Input: dimensioned drawing with shaded views. Units: mm. Origin: part minimum x, y, z. A direction names the side the tool comes from. Round coordinates to 2 decimals unless told otherwise and drop trailing zeros. Loops run counter-clockwise (first coordinate to the right, second up) from the corner with the lowest first, then second, coordinate; pieces in that order, holes last. Notation, with made-up numbers: M 39,-32 L 80,-32 A25 cw 80,0 Z; hole C 23.25,-11.75 d11. An arc over 180 degrees is marked long. Answer as a JSON object with one key per item and string values.
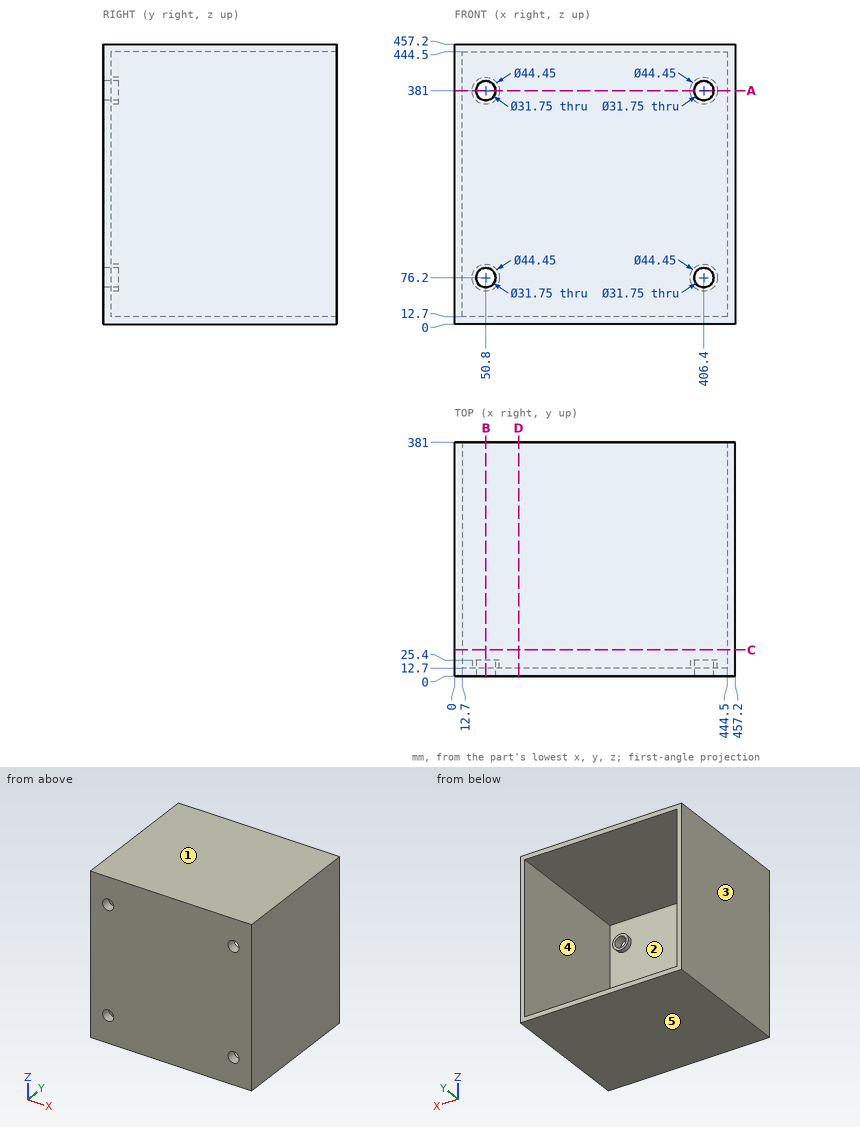
Item 1: Access query for the marked faces 1 and 2. Directions: +Z, -Z, +X, -X, +Y, -Y. A direction counts if a zero-diameter tool reaches every point of the face in a straight line with its end or side. Return the directions, or none.
Answer sheet:
{"face 1": "+Z, +X, -X, +Y, -Y", "face 2": "+Y"}
Item 2: Section B-B on x = 50.8. Return the cut outline in (y, z) (3 decimals), then the cut area to 3 significant figures.
Answer sheet:
{"outline": "M 0,0 L 381,0 L 381,12.7 L 12.7,12.7 L 12.7,53.975 L 25.4,53.975 L 25.4,60.325 L 0,60.325 Z; M 0,92.075 L 25.4,92.075 L 25.4,98.425 L 12.7,98.425 L 12.7,358.775 L 25.4,358.775 L 25.4,365.125 L 0,365.125 Z; M 0,396.875 L 25.4,396.875 L 25.4,403.225 L 12.7,403.225 L 12.7,444.5 L 381,444.5 L 381,457.2 L 0,457.2 Z", "area": "14,700 mm²"}
Item 3: Pull-direction query (X, two-part tool) for the marked faces 3, 4 and 5; classes: pulls with the +X half, pulls with the -X half, needs draft (parallel to the pull), parting line crosses it, or undercut.
Answer sheet:
{"face 3": "pulls with the -X half", "face 4": "undercut", "face 5": "needs draft"}
Item 4: Line query: probe 1 along Z at (x, y) = (406, 16); probe 2 along X at (y, z) = (11.75, 381) (3 decimals); probe 3 along X at (y, z) = (18, 381) (3 decimals). Output: solid intervals per line, ascending. Write a range as from..to.
Answer sheet:
{"probe 1": "z = 0..12.7, 53.98..60.33, 92.07..98.42, 358.78..365.13, 396.87..403.22, 444.5..457.2", "probe 2": "x = 0..34.925, 66.675..390.525, 422.275..457.2", "probe 3": "x = 0..12.7, 28.575..34.925, 66.675..73.025, 384.175..390.525, 422.275..428.625, 444.5..457.2"}
Item 5: Contact query for flat-ended pins moving along their axis: pin 1 Ø8 at (x, z) = (285.5, 287.5) entering from +Y; pin 2 Ø13.5 at (x, z) = (398.5, 66) entering from +Y. Output: stop coordinate, or through.
Answer sheet:
{"pin 1": "stops at y = 12.7", "pin 2": "stops at y = 25.4"}
Item 6: Section D-D on x = 104.5. Return the cut outline in (y, z).
Answer sheet:
{"outline": "M 0,0 L 381,0 L 381,12.7 L 12.7,12.7 L 12.7,444.5 L 381,444.5 L 381,457.2 L 0,457.2 Z"}
Item 7: Section C-C on y = 42.5. Return the cut outline in (x, z).
Answer sheet:
{"outline": "M 0,0 L 457.2,0 L 457.2,457.2 L 0,457.2 Z; hole M 12.7,12.7 L 444.5,12.7 L 444.5,444.5 L 12.7,444.5 Z"}
Item 8: Section A-A on z = 381. Return the cut outline in (x, y) (3 decimals), then the cut area to 3 significant figures.
Answer sheet:
{"outline": "M 0,0 L 34.925,0 L 34.925,25.4 L 28.575,25.4 L 28.575,12.7 L 12.7,12.7 L 12.7,381 L 0,381 Z; M 66.675,0 L 390.525,0 L 390.525,25.4 L 384.175,25.4 L 384.175,12.7 L 73.025,12.7 L 73.025,25.4 L 66.675,25.4 Z; M 422.275,0 L 457.2,0 L 457.2,381 L 444.5,381 L 444.5,12.7 L 428.625,12.7 L 428.625,25.4 L 422.275,25.4 Z", "area": "14,700 mm²"}
